The model under review builds one solid part; all positions refer to its coordinate system, in mm. Give positions to 0.01 mm unless a question says otherwise; leave off trailing zeros. Answer as a JSON object with one key per item and string values. Group by question number.
from build123d import *

# Parameters (mm, degrees)
PAD_DEPTH       = 25
FILLET_R        = 24
POCKET_DEPTH    = 100
POCKET001_DEPTH = 15


with BuildPart() as part:
    # Sketch → Pad (new body)
    with BuildSketch(Plane.XY):
        with BuildLine():
            ThreePointArc((-25, 25), (-50, 0), (-25, -25))
            Line((-25, -25), (25, -25))
            ThreePointArc((25, -25), (50, 0), (25, 25))
            Line((-25, 25), (25, 25))
        make_face()
    extrude(amount=PAD_DEPTH)

    # Fillet
    fillet_edges = [part.edges().sort_by_distance(p)[0] for p in [
        (0, 25, 25),
    ]]
    fillet(fillet_edges, radius=FILLET_R)

    # Sketch001 → Pocket (cut)
    with BuildSketch(Plane.YZ.offset(50)):
        Polygon((-25, 1), (0, 26), (-25, 26), align=None)
    extrude(amount=-POCKET_DEPTH, mode=Mode.SUBTRACT)

    # Sketch002 → Pocket001 (cut)
    with BuildSketch(Plane.XY.offset(25)):
        with BuildLine():
            Line((-50, 5), (-50, 6))
            add(Edge.make_bspline(
                [(-50, 6), (0, 21), (50, 6)],
                knots=[0, 0, 0, 1, 1, 1], degree=2))
            Line((50, 6), (50, 5))
            add(Edge.make_bspline(
                [(-50, 5), (0, 20), (50, 5)],
                knots=[0, 0, 0, 1, 1, 1], degree=2))
        make_face()
    extrude(amount=-POCKET001_DEPTH, mode=Mode.SUBTRACT)


solid = part.part
1. For pin 1 (2 mm diameter, centred on x = -6, z = 7.5, fed in from -Y); pin 2 (2 mm diameter, centred on x = -27.5, z = 10.5, fed in from -Y); pin 3 (4 mm diameter, centred on x = -2, y = 8.5, fed in from +Z), all flat-tipped, find the tip position at first contact; note any pin that passes through.
2. For probe 1 along Y at (x, z) = (-6.5, 15.5); probe 2 along Y at (x, z) = (12.5, 21.25); probe 3 along Y at (x, z) = (-34, 4.75), list the stretches that pass through material, from the lowest coordinate up. Write a range as [from, to].
3. Draft analysis for pull direction Y (two halves, no side actions). For faces 1 (the flat face through (0, 13, 10)), 2 (the cylindrical face through (0.35, 7.016, 24.234)), 3 (the flat face through (1, -13, 13)), 4 (the cylindrical face through (-49.994, 0.55, 0.493)), state which applies: pulls with the +Y half, pulls with the -Y half, needs draft (parallel to the pull), parting line crosses it, or undercut.
Checks:
{
 "1": {"pin 1": "stops at y = -19.5", "pin 2": "stops at y = -16.5", "pin 3": "stops at z = 24.36"},
 "2": {"probe 1": "y = [-10.5, 12.37], [13.37, 20.12]", "probe 2": "y = [-4.75, 12.03], [13.03, 13.88]", "probe 3": "y = [-21.25, 23.01]"},
 "3": {"face 1": "undercut", "face 2": "pulls with the +Y half", "face 3": "pulls with the -Y half", "face 4": "parting line crosses it"}
}
